from build123d import *

# Parameters (mm, degrees)
F0_R     = 6
F1_DEPTH = 5


with BuildPart() as f1:
    # F0 (on Top) → F1 (new body)
    with BuildSketch(Plane.XY):
        with Locations((0.1191368553, 0.0803260972)):
            Circle(F0_R)
        with BuildLine():
            ThreePointArc((4.2675466454, 1.8240853161), (4.3988911787, 1.4709025719), (4.5002268275, 1.1079693501))
            ThreePointArc((4.5002268275, 1.1079693501), (5.3073148215, 0.8527258233), (5.6536368553, 0.0803260972))
            ThreePointArc((5.6536368553, 0.0803260972), (5.3073148215, -0.6920736289), (4.5002268275, -0.9473171557))
            ThreePointArc((4.5002268275, -0.9473171557), (4.3988911787, -1.3102503775), (4.2675466454, -1.6634331217))
            ThreePointArc((4.2675466454, -1.6634331217), (4.6528941109, -2.0427704321), (4.79421333, -2.5647075381))
            ThreePointArc((4.79421333, -2.5647075381), (4.1755248273, -3.5119620175), (3.059479548, -3.3261948332))
            ThreePointArc((3.059479548, -3.3261948332), (2.7641704906, -3.5602503775), (2.4503149228, -3.76877884))
            ThreePointArc((2.4503149228, -3.76877884), (2.5204661677, -3.9790445807), (2.54421333, -4.1994282261))
            ThreePointArc((2.54421333, -4.1994282261), (1.6124558319, -5.2288135905), (0.4956212985, -4.4038972987))
            ThreePointArc((0.4956212985, -4.4038972987), (0.1191368553, -4.4196739028), (-0.2573475879, -4.4038972987))
            ThreePointArc((-0.2573475879, -4.4038972987), (-1.5911177, -5.1832961922), (-2.2120412121, -3.76877884))
            ThreePointArc((-2.2120412121, -3.76877884), (-2.52589678, -3.5602503775), (-2.8212058374, -3.3261948332))
            ThreePointArc((-2.8212058374, -3.3261948332), (-4.3583677, -3.1727713816), (-4.0292729348, -1.6634331217))
            ThreePointArc((-4.0292729348, -1.6634331217), (-4.160617468, -1.3102503775), (-4.2619531169, -0.9473171557))
            ThreePointArc((-4.2619531169, -0.9473171557), (-5.4153631447, 0.0803260972), (-4.2619531169, 1.1079693501))
            ThreePointArc((-4.2619531169, 1.1079693501), (-4.160617468, 1.4709025719), (-4.0292729348, 1.8240853161))
            ThreePointArc((-4.0292729348, 1.8240853161), (-4.3583677, 3.333423576), (-2.8212058374, 3.4868470276))
            ThreePointArc((-2.8212058374, 3.4868470276), (-2.52589678, 3.7209025719), (-2.2120412121, 3.9294310345))
            ThreePointArc((-2.2120412121, 3.9294310345), (-1.5911177, 5.3439483866), (-0.2573475879, 4.5645494931))
            ThreePointArc((-0.2573475879, 4.5645494931), (0.1191368553, 4.5803260972), (0.4956212985, 4.5645494931))
            ThreePointArc((0.4956212985, 4.5645494931), (1.6124558319, 5.3894657849), (2.54421333, 4.3600804205))
            ThreePointArc((2.54421333, 4.3600804205), (2.5204661677, 4.1396967751), (2.4503149228, 3.9294310345))
            ThreePointArc((2.4503149228, 3.9294310345), (2.7641704906, 3.7209025719), (3.059479548, 3.4868470276))
            ThreePointArc((3.059479548, 3.4868470276), (4.1755248273, 3.6726142119), (4.79421333, 2.7253597325))
            ThreePointArc((4.79421333, 2.7253597325), (4.6528941109, 2.2034226265), (4.2675466454, 1.8240853161))
        make_face(mode=Mode.SUBTRACT)
        with BuildLine():
            ThreePointArc((4.5002268275, -0.9473171557), (4.5893105027, -0.4369239028), (4.6191368553, 0.0803260972))
            ThreePointArc((4.6191368553, 0.0803260972), (4.5893105027, 0.5975760972), (4.5002268275, 1.1079693501))
            ThreePointArc((4.5002268275, 1.1079693501), (3.5846368553, 0.0803260972), (4.5002268275, -0.9473171557))
        make_face()
        with BuildLine():
            ThreePointArc((4.5002268275, 1.1079693501), (4.5893105027, 0.5975760972), (4.6191368553, 0.0803260972))
            ThreePointArc((4.6191368553, 0.0803260972), (4.5893105027, -0.4369239028), (4.5002268275, -0.9473171557))
            ThreePointArc((4.5002268275, -0.9473171557), (5.3073148215, -0.6920736289), (5.6536368553, 0.0803260972))
            ThreePointArc((5.6536368553, 0.0803260972), (5.3073148215, 0.8527258233), (4.5002268275, 1.1079693501))
        make_face()
        with BuildLine():
            ThreePointArc((3.059479548, 3.4868470276), (2.9227852493, 2.117295889), (4.2675466454, 1.8240853161))
            ThreePointArc((4.2675466454, 1.8240853161), (3.75971333, 2.7253597325), (3.059479548, 3.4868470276))
        make_face()
        with BuildLine():
            ThreePointArc((3.059479548, 3.4868470276), (3.75971333, 2.7253597325), (4.2675466454, 1.8240853161))
            ThreePointArc((4.2675466454, 1.8240853161), (4.6528941109, 2.2034226265), (4.79421333, 2.7253597325))
            ThreePointArc((4.79421333, 2.7253597325), (4.1755248273, 3.6726142119), (3.059479548, 3.4868470276))
        make_face()
        with BuildLine():
            ThreePointArc((4.79421333, -2.5647075381), (4.6528941109, -2.0427704321), (4.2675466454, -1.6634331217))
            ThreePointArc((4.2675466454, -1.6634331217), (3.75971333, -2.5647075381), (3.059479548, -3.3261948332))
            ThreePointArc((3.059479548, -3.3261948332), (4.1755248273, -3.5119620175), (4.79421333, -2.5647075381))
        make_face()
        with BuildLine():
            ThreePointArc((3.059479548, -3.3261948332), (3.75971333, -2.5647075381), (4.2675466454, -1.6634331217))
            ThreePointArc((4.2675466454, -1.6634331217), (2.9227852493, -1.9566436946), (3.059479548, -3.3261948332))
        make_face()
        with BuildLine():
            ThreePointArc((0.4956212985, 4.5645494931), (1.1900352493, 3.3762124544), (2.4503149228, 3.9294310345))
            ThreePointArc((2.4503149228, 3.9294310345), (1.50971333, 4.3600804205), (0.4956212985, 4.5645494931))
        make_face()
        with BuildLine():
            ThreePointArc((0.4956212985, 4.5645494931), (1.50971333, 4.3600804205), (2.4503149228, 3.9294310345))
            ThreePointArc((2.4503149228, 3.9294310345), (2.5204661677, 4.1396967751), (2.54421333, 4.3600804205))
            ThreePointArc((2.54421333, 4.3600804205), (1.6124558319, 5.3894657849), (0.4956212985, 4.5645494931))
        make_face()
        with BuildLine():
            ThreePointArc((2.54421333, -4.1994282261), (2.5204661677, -3.9790445807), (2.4503149228, -3.76877884))
            ThreePointArc((2.4503149228, -3.76877884), (1.50971333, -4.1994282261), (0.4956212985, -4.4038972987))
            ThreePointArc((0.4956212985, -4.4038972987), (1.6124558319, -5.2288135905), (2.54421333, -4.1994282261))
        make_face()
        with BuildLine():
            ThreePointArc((0.4956212985, -4.4038972987), (1.50971333, -4.1994282261), (2.4503149228, -3.76877884))
            ThreePointArc((2.4503149228, -3.76877884), (1.1900352493, -3.21556026), (0.4956212985, -4.4038972987))
        make_face()
        with BuildLine():
            ThreePointArc((-0.2369396194, 4.3600804205), (-0.242054255, 4.4628229225), (-0.2573475879, 4.5645494931))
            ThreePointArc((-0.2573475879, 4.5645494931), (-1.2714396194, 4.3600804205), (-2.2120412121, 3.9294310345))
            ThreePointArc((-2.2120412121, 3.9294310345), (-1.051055974, 3.3493275829), (-0.2369396194, 4.3600804205))
        make_face()
        with BuildLine():
            ThreePointArc((-2.2120412121, 3.9294310345), (-1.2714396194, 4.3600804205), (-0.2573475879, 4.5645494931))
            ThreePointArc((-0.2573475879, 4.5645494931), (-1.5911177, 5.3439483866), (-2.2120412121, 3.9294310345))
        make_face()
        with BuildLine():
            ThreePointArc((-2.2120412121, -3.76877884), (-1.5911177, -5.1832961922), (-0.2573475879, -4.4038972987))
            ThreePointArc((-0.2573475879, -4.4038972987), (-1.2714396194, -4.1994282261), (-2.2120412121, -3.76877884))
        make_face()
        with BuildLine():
            ThreePointArc((-2.2120412121, -3.76877884), (-1.2714396194, -4.1994282261), (-0.2573475879, -4.4038972987))
            ThreePointArc((-0.2573475879, -4.4038972987), (-0.242054255, -4.302170728), (-0.2369396194, -4.1994282261))
            ThreePointArc((-0.2369396194, -4.1994282261), (-1.051055974, -3.1886753885), (-2.2120412121, -3.76877884))
        make_face()
        with BuildLine():
            ThreePointArc((-2.4869396194, 2.7253597325), (-2.57418514, 3.1411712298), (-2.8212058374, 3.4868470276))
            ThreePointArc((-2.8212058374, 3.4868470276), (-3.5214396194, 2.7253597325), (-4.0292729348, 1.8240853161))
            ThreePointArc((-4.0292729348, 1.8240853161), (-2.9995025134, 1.8321789516), (-2.4869396194, 2.7253597325))
        make_face()
        with BuildLine():
            ThreePointArc((-4.0292729348, 1.8240853161), (-3.5214396194, 2.7253597325), (-2.8212058374, 3.4868470276))
            ThreePointArc((-2.8212058374, 3.4868470276), (-4.3583677, 3.333423576), (-4.0292729348, 1.8240853161))
        make_face()
        with BuildLine():
            ThreePointArc((-4.0292729348, -1.6634331217), (-4.3583677, -3.1727713816), (-2.8212058374, -3.3261948332))
            ThreePointArc((-2.8212058374, -3.3261948332), (-3.5214396194, -2.5647075381), (-4.0292729348, -1.6634331217))
        make_face()
        with BuildLine():
            ThreePointArc((-4.0292729348, -1.6634331217), (-3.5214396194, -2.5647075381), (-2.8212058374, -3.3261948332))
            ThreePointArc((-2.8212058374, -3.3261948332), (-2.57418514, -2.9805190354), (-2.4869396194, -2.5647075381))
            ThreePointArc((-2.4869396194, -2.5647075381), (-2.9995025134, -1.6715267572), (-4.0292729348, -1.6634331217))
        make_face()
        with BuildLine():
            ThreePointArc((-3.3463631447, 0.0803260972), (-3.6084634186, 0.7685040634), (-4.2619531169, 1.1079693501))
            ThreePointArc((-4.2619531169, 1.1079693501), (-4.3808631447, 0.0803260972), (-4.2619531169, -0.9473171557))
            ThreePointArc((-4.2619531169, -0.9473171557), (-3.6084634186, -0.607851869), (-3.3463631447, 0.0803260972))
        make_face()
        with BuildLine():
            ThreePointArc((-4.2619531169, -0.9473171557), (-4.3808631447, 0.0803260972), (-4.2619531169, 1.1079693501))
            ThreePointArc((-4.2619531169, 1.1079693501), (-5.4153631447, 0.0803260972), (-4.2619531169, -0.9473171557))
        make_face()
    extrude(amount=F1_DEPTH)


solid = f1.part
Source: CAD feature listing. Evaluate the final solid. Frame: model axes, mm. Coordinates: 2 decimals unless noted, no trailing zeros. Loops run counter-clockwise (first coordinate to the right, second up) from the corner with the lowest first, then second, coordinate; pieces in that order, holes last. Notation, with made-up numbers: (38, 46.25) - (56, 46.25) arc R25 cw to (56, 69.25) - close; hole circle Ø1 at (-8, -34). An arc over 180 degrees is marked (long way). One line per question, with ' | ' between items.
1) Section C-C, the plane y = 0.5. Return loops of the section in (x, z), then the cut area to 3 significant figures.
Report:
outline: (-5.87, 0) - (-3.44, 0) - (-3.44, 5) - (-5.87, 5) - close; (3.67, 0) - (6.1, 0) - (6.1, 5) - (3.67, 5) - close | area: 24.3 mm²
2) Section D-D, the plane x = 5.25. Return loops of the section in (y, z).
Report:
outline: (-3.03, 0) - (3.19, 0) - (3.19, 5) - (-3.03, 5) - close
3) Line query: line 1 along Y through (x, z) = (-4, 4.25); line 2 along X through (y, z) = (-0.75, 4.2); line 3 along Y through (x, z) = (2, 1.55). Output: solid intervals per line, ascending.
Report:
line 1: y = -4.28 to -1.65, -0.88 to 1.04, 1.81 to 4.44 | line 2: x = -5.82 to -3.76, 4 to 6.06 | line 3: y = -5.62 to -3.29, 3.45 to 5.78
4) First-contact query: P1, Ø1, axis at y = -4.5, z = 1, coming from the +X side. Flat tip, straight axial feed; report the tip coordinate or a pass-through.
Report:
P1: stops at x = 4.52
5) Pull-direction query (Y, two-part tool) for faces 1 (the face through (1.17, 3.383, 2.465)), 2 (the face through (-3, -3, 5)), 3 (the face through (5.842, 1.883, 2.465)); classes: released by +Y, released by -Y, zero draft, split by the parting line, or undercut.
Report:
face 1: undercut | face 2: zero draft | face 3: split by the parting line
6) Section A-A, the plane x = -1.75. Return loops of the section in (y, z).
Report:
outline: (-5.62, 0) - (-3.28, 0) - (-3.28, 5) - (-5.62, 5) - close; (3.44, 0) - (5.78, 0) - (5.78, 5) - (3.44, 5) - close
